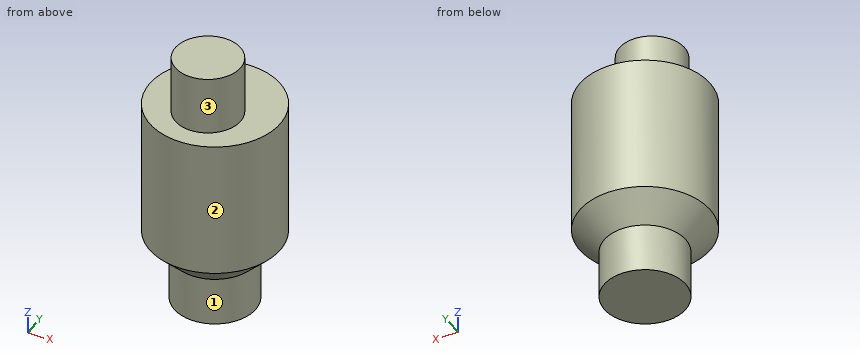
from build123d import *

# Parameters (mm, degrees)
CYLINDER_R             = 2
CYLINDER_DEPTH         = 5
CHAMFER_SIZE           = 0.75
CYLINDER002_R          = 1
CYLINDER002_DEPTH      = 1.8
CYLINDER001_R          = 1.25
CYLINDER001_DEPTH      = 1.5
FUSION_PLACEMENT_ANGLE = 180


with BuildPart() as chamfer001:
    # Cylinder → Cylinder (new body)
    with BuildSketch(Plane.XY):
        Circle(CYLINDER_R)
    extrude(amount=CYLINDER_DEPTH)

    # Chamfer
    chamfer_edges = [chamfer001.edges().sort_by_distance(p)[0] for p in [
        (-2, 0, 5),
    ]]
    chamfer(chamfer_edges, length=CHAMFER_SIZE)


with BuildPart() as chamfer001_1:
    # Clone002 placement: moved
    add(chamfer001.part.moved(Location((0, -6, 0))))


with BuildPart() as cylinder004:
    # Cylinder002 → Cylinder002 (new body)
    with BuildSketch(Plane.XY.offset(-1.8)):
        Circle(CYLINDER002_R)
    extrude(amount=CYLINDER002_DEPTH)


with BuildPart() as cylinder004_1:
    # Clone001 placement: moved
    add(cylinder004.part.moved(Location((0, -6.4, 0))))


with BuildPart() as obj1:
    # Cylinder001 → Cylinder001 (new body)
    with BuildSketch(Plane.XY.offset(5)):
        Circle(CYLINDER001_R)
    extrude(amount=CYLINDER001_DEPTH)


with BuildPart() as obj1_1:
    # Clone placement: moved
    add(obj1.part.moved(Location((0, -6, 0))))

    # Fusion: union Chamfer001, Cylinder004
    add(chamfer001_1.part)
    add(cylinder004_1.part)


with BuildPart() as obj1_2:
    # Fusion placement: moved
    add(obj1_1.part.moved(Location((-45, 65, 6.5))).rotate(Axis((-45, 65, 6.5), (0, 1, 0)), FUSION_PLACEMENT_ANGLE))


solid = obj1_2.part
Can you work these out from the model? Positions are in its coordinate system, mm. Face numbers are marked on the shaded views. A direction names the side the tool comes from. Give positions to 0.01 mm unless a question says otherwise; leave off trailing zeros. Loops run counter-clockwise (first coordinate to the right, second up) from the corner with the lowest first, then second, coordinate; pieces in that order, holes last. Notation, with made-up numbers: (28.25, 10.25) -> (54.25, 10.25) arc R19 ccw to (54.25, 44.25) -> close; hole circle Ø11 at (-37, 77.25). An arc over 180 degrees is marked (long way). Return JSON: item names as keys, results as strings.
Q1. I want a section at D-D, the plane z = 5. List the corners of the cut face in (x, y) for me.
Checks:
{"outline": "circle Ø4 at (-45, 59)"}
Q2. I want a section at B-B, the plane y = 59. List the corners of the cut face in (x, z) for me.
Checks:
{"outline": "(-47, 2.25) -> (-46.25, 1.5) -> (-46.25, 0) -> (-43.75, 0) -> (-43.75, 1.5) -> (-43, 2.25) -> (-43, 6.5) -> (-44.08, 6.5) -> (-44.08, 8.3) -> (-45.92, 8.3) -> (-45.92, 6.5) -> (-47, 6.5) -> close"}
Q3. I need wall thicknesses on probe 1 along Z at (x, y) = (-44.3, 59.95); probe 2 along Z at (x, y) = (-45.1, 60.65); probe 3 along Y at (x, z) = (-46, 6). Which ranges of each line are inside material? Lowest first, please.
Checks:
{"probe 1": "z = 0 to 6.5", "probe 2": "z = 1.9 to 6.5", "probe 3": "y = 57.27 to 60.73"}
Q4. On a 3-axis mill with a long thin cutter (end or side, diameter ignored), from which of +Z, -Z, +X, -X, +Y, -Y can I reach the whole of each face in a straight line? I mean the marked faces 1, 2 and 3. Say none if no direction works.
Checks:
{"face 1": "-Z", "face 2": "+Z, -Z", "face 3": "+Z"}
Q5. I want a section at C-C, the plane z = 0.5. List the corners of the cut face in (x, y) for me.
Checks:
{"outline": "circle Ø2.5 at (-45, 59)"}
Q6. I want a section at A-A, the plane x = -45. List the corners of the cut face in (y, z) for me, then the cut area to 3 significant figures.
Checks:
{"outline": "(57, 2.25) -> (57.75, 1.5) -> (57.75, 0) -> (60.25, 0) -> (60.25, 1.5) -> (61, 2.25) -> (61, 6.5) -> (59.6, 6.5) -> (59.6, 8.3) -> (57.6, 8.3) -> (57.6, 6.5) -> (57, 6.5) -> close", "area": "26.8 mm2"}
Q7. For pin 1 Ø2 at (x, z) = (-46.5, 4) entering from -Y; pin 2 Ø1.5 at (x, z) = (-46.5, 7) entering from -Y, each with a flat end and sliding along its axis, tell me the tip position at first contact or that it passes through.
Checks:
{"pin 1": "stops at y = 57.06", "pin 2": "stops at y = 57.24"}
